Input: part model. Units: mm. Frame: model coordinates. Face numbers are marked on the shaded views. A direction names the side the tool comes from. Round coordinates to 2 decimals unless told otherwise and drop trailing zeros. Loops run counter-clockwise (first coordinate to the right, second up) from the corner with the lowest first, then second, coordinate; pieces in that order, holes last. Notation, with made-up numbers: M 26,-23 L 46,-23 A11 ccw 46,-11 Z; hole C 79,73 d10. An arc over 180 degrees is marked long. Use one line per item in the form item = value. Start each with the question number.
Q1. First-contact query: P1, Ø3.5, axis at x = 0, y = 0, coming from the -Z side; P2, Ø2, axis at x = 4, z = 1, coming from the -Y side; P3, Ø3, axis at y = 3, z = 2.5, coming from the +X side; P4, Ø3, axis at x = -3.5, z = 3.5, coming from the -Y side. Flat tips, straight axial feed; report the tip coordinate or a pass-through.
Q2. Mould query, pull axis X, two halves, no side actions, for the marked faces 4, 5 and 6. Classes: pulls with the +X half, pulls with the -X half, needs draft (parallel to the pull), parting line crosses it, or undercut.
Q3. Section query A-A, the plane z = 2.5. Output: boundary loops of the cut face in (x, y).
Q4. Ray query, line 1 along Y through (x, z) = (0, 0.4) (3 decimals); line 2 along Y through (x, z) = (0.5, 4.7); line 3 along Y through (x, z) = (0.25, 3.75). Return the intervals inside material, ascending.
Q5. Access query for the marked faces 1, 2 and 3. Directions: +Z, -Z, +X, -X, +Y, -Y. A direction counts if a zero-diameter tool reaches every point of the face in a straight line with its end or side. Return the directions, or none.
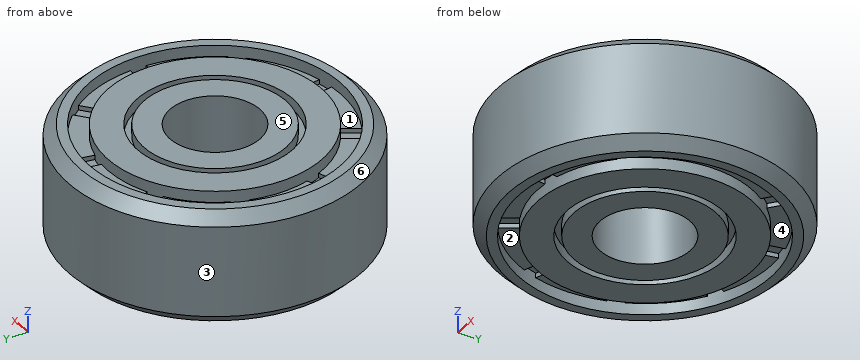
Autodesk Inventor part; units mm, degrees
ref_plane "Work Plane1" through (0, 0, 2.5) normal (0, 0, -1) x (-1, 0, 0)
ref_plane "YZ Plane" through (0, 0, 0) normal (1, 0, 0) x (0, 1, 0)
ref_plane "XZ Plane" through (0, 0, 0) normal (0, 1, 0) x (-1, 0, 0)
sketch "Sketch1" plane through (0, 0, 0) normal (0, 0, 1) x (1, 0, 0)
  circle A0 centre (0, 0) radius 6.5
  circle A1 centre (0, 0) radius 2
  dimension "d0" = 13
  dimension "d1" = 4
extrude "Extrusion1" add sketch "Sketch1" along normal blind 5
chamfer "Chamfer1" distance 0.5 angle 45 2 edges at (-6.5, 0, 5) (-6.5, 0, 0)
sketch "Sketch2" plane through (0, 0, 5) normal (0, 0, 1) x (1, 0, 0)
  circle A0 centre (0, 0) radius 6
  circle A1 centre (0, 0) radius 3.15
  circle A2 centre (0, 0) radius 3.45
  circle A3 centre (0, 0) radius 4.75
  circle A4 centre (0, 0) radius 5.575
  dimension "d7" = 6.3
  dimension "d8" = 6.9
  dimension "d9" = 9.5
  dimension "d10" = 11.15
extrude "Extrusion2" cut sketch "Sketch2" against normal blind 0.5 contours A2 | A4
ref_plane "Work Plane1" through (0, 0, 2.5) normal (0, 0, -1) x (-1, 0, 0)
sketch "Sketch3" plane through (0, 0, 4.5) normal (0, 0, 1) x (1, 0, 0)
  circle A0 centre (0, 0) radius 4.75
  circle A1 centre (0, 0) radius 5.575
  circle A2 centre (0, 0) radius 4.75 construction
  circle A3 centre (0, 0) radius 5.575 construction
  line L0 (-9.1, 0) -> (9.1, 0) construction
  line L1 (4.6568, 0.35) -> (5.7132, 0.35)
  line L2 (4.5944, -0.35) -> (5.8021, -0.35)
  line L3 (5.349, 0.35) -> (5.7285, 0.35)
  arc A4 (4.7371, -0.35) -> (4.7371, 0.35) centre (0, 0) ccw
  arc A5 (5.564, -0.35) -> (5.564, 0.35) centre (0, 0) ccw
  dimension "d14" = 0.35
  dimension "d15" = 0.35
extrude "Extrusion3" cut sketch "Sketch3" against normal blind 0.2 contours A0 L1 A1 L2 picked at (5.2247, 0.1167)
pattern_circular "Circular Pattern1" count 9 over 360 about axis through (0, 0, -10) along (0, 0, 1) of "Extrusion3"
mirror "Mirror1" about plane through (0, 0, 2.5) normal (0, 0, -1) of "Circular Pattern1", "Extrusion2"
properties part number "Bearing-605zz" material "Stainless Steel"
Results found:
q1.P1 = through
q1.P2 = -5.77
q1.P3 = 6.32
q1.P4 = -6.18
q2.face_4 = undercut
q2.face_5 = needs draft
q2.face_6 = parting line crosses it
q3.outline = C 0,0 d13; hole C 0,0 d4
q4.line_1 = -6.4 to -5.575, -4.75 to -3.45, -3.15 to -2, 2 to 3.15, 3.45 to 4.75, 5.575 to 6.4
q4.line_2 = -6.28 to -5.55, -4.72 to -3.41, -3.11 to -1.94, 1.94 to 3.11, 3.41 to 4.72, 5.55 to 6.28
q4.line_3 = -6.5 to -1.98, 1.98 to 6.5
q5.face_1 = +Z
q5.face_2 = -Z
q5.face_3 = +Z, -Z
